```python
from build123d import *

# Parameters (mm, degrees)
SKETCH1_W           = 210
SKETCH1_H           = 439.61
BOSS_EXTRUDE1_DEPTH = 2
SKETCH2_W           = 210
SKETCH2_H           = 2
BOSS_EXTRUDE2_DEPTH = 20.32
FILLET1_R           = 1
FILLET2_R           = 1.5
SKETCH4_R           = 1.6
CUT_EXTRUDE1_DEPTH  = 1134.166859304


with BuildPart() as part:
    # Sketch1 → Boss-Extrude1 (new body)
    with BuildSketch(Plane(origin=(0, 0, 0), x_dir=(1, 0, 0), z_dir=(0, 1, 0))):
        with Locations((988.720815229, 75.734721456)):
            Rectangle(SKETCH1_W, SKETCH1_H)
    extrude(amount=BOSS_EXTRUDE1_DEPTH)

    # Sketch2 → Boss-Extrude2 (add)
    with BuildSketch(Plane.XZ):
        with Locations((988.720815229, 143.070278544)):
            Rectangle(SKETCH2_W, SKETCH2_H)
        with Locations((988.720815229, -294.539721456)):
            Rectangle(SKETCH2_W, SKETCH2_H)
    extrude(amount=BOSS_EXTRUDE2_DEPTH)

    # Fillet1
    fillet1_edges = [part.edges().sort_by_distance(p)[0] for p in [
        (988.720815229, 0, 142.070278544),
        (988.720815229, 0, -293.539721456),
    ]]
    fillet(fillet1_edges, radius=FILLET1_R)

    # Fillet2
    fillet2_edges = [part.edges().sort_by_distance(p)[0] for p in [
        (988.720815229, 2, 144.070278544),
        (988.720815229, 2, -295.539721456),
    ]]
    fillet(fillet2_edges, radius=FILLET2_R)

    # Sketch4 → Cut-Extrude1 (cut, through all)
    with BuildSketch(Plane(origin=(0, 2, 0), x_dir=(1, 0, 0), z_dir=(0, 1, 0))):
        with Locations(Location((921.920815229, 214.039721456, 0), (0, 0, 270))):
            Circle(SKETCH4_R)
        with Locations(Location((921.920815229, 274.039721456, 0), (0, 0, 270))):
            Circle(SKETCH4_R)
        with Locations(Location((986.920815229, 234.750399575, 0), (0, 0, 270))):
            Circle(SKETCH4_R)
        with Locations(Location((986.920815229, 274.039721456, 0), (0, 0, 270))):
            Circle(SKETCH4_R)
        with Locations(Location((1010.309162877, 65.651373808, 0), (0, 0, 270))):
            Circle(SKETCH4_R)
        with Locations(Location((1010.309162877, 95.651373808, 0), (0, 0, 270))):
            Circle(SKETCH4_R)
        with Locations(Location((986.565606348, -21.848626192, 0), (0, 0, 270))):
            Circle(SKETCH4_R)
        with Locations(Location((959.065606348, -21.848626192, 0), (0, 0, 270))):
            Circle(SKETCH4_R)
        with Locations(Location((963.168146726, 43.151373808, 0), (0, 0, 270))):
            Circle(SKETCH4_R)
        with Locations(Location((921.565606348, 43.151373808, 0), (0, 0, 270))):
            Circle(SKETCH4_R)
        with Locations(Location((894.065606348, -34.348626192, 0), (0, 0, 270))):
            Circle(SKETCH4_R)
        with Locations(Location((894.065606348, 15.651373808, 0), (0, 0, 270))):
            Circle(SKETCH4_R)
        with Locations(Location((961.370669454, -59.263980407, 0), (0, 0, 270))):
            Circle(SKETCH4_R)
        with Locations(Location((945.453731167, -122.879875269, 0), (0, 0, 270))):
            Circle(SKETCH4_R)
        with Locations(Location((896.92248209, -74.348626192, 0), (0, 0, 270))):
            Circle(SKETCH4_R)
        with Locations(Location((1073.720815229, -60.736751011, 0), (0, 0, 270))):
            Circle(SKETCH4_R)
        with Locations(Location((985.453731167, -60.736751011, 0), (0, 0, 270))):
            Circle(SKETCH4_R)
        with Locations(Location((1073.720815229, -125.736751011, 0), (0, 0, 270))):
            Circle(SKETCH4_R)
        with Locations(Location((985.453731167, -125.736751011, 0), (0, 0, 270))):
            Circle(SKETCH4_R)
        with Locations(Location((1013.305977837, -13.343657344, 0), (0, 0, 270))):
            Circle(SKETCH4_R)
        with Locations(Location((1058.564216667, 12.786773537, 0), (0, 0, 270))):
            Circle(SKETCH4_R)
        with Locations(Location((996.746475218, 52.151079456, 0), (0, 0, 270))):
            Circle(SKETCH4_R)
        with Locations(Location((938.352910915, 174.501024052, 0), (0, 0, 270))):
            Circle(SKETCH4_R)
        with Locations(Location((998.456987316, 114.396947651, 0), (0, 0, 270))):
            Circle(SKETCH4_R)
        with Locations(Location((998.866251712, 205.91156481, 0), (0, 0, 270))):
            Circle(SKETCH4_R)
        with Locations(Location((1058.970328113, 145.807488409, 0), (0, 0, 270))):
            Circle(SKETCH4_R)
        with Locations(Location((1075.308219227, 106.361698083, 0), (0, 0, 270))):
            Circle(SKETCH4_R)
        with Locations(Location((1075.305408117, 46.781698149, 0), (0, 0, 270))):
            Circle(SKETCH4_R)
    extrude(amount=-CUT_EXTRUDE1_DEPTH, mode=Mode.SUBTRACT)


solid = part.part
```
Can you work these out from the model? Positions are in its coordinate system, mm. A direction names the side the tool comes from. Coordinates: 2 decimals unless noted, no trailing zeros. Loops run counter-clockwise (first coordinate to the right, second up) from the corner with the lowest first, then second, coordinate; pieces in that order, holes last. Notation, with made-up numbers: (26.25, 81.5) -> (55.25, 81.5) arc R22 cw to (55.25, 105.5) -> close; hole circle Ø10 at (13, 78.5). An arc over 180 degrees is marked (long way). Answer as a JSON object with one key per item and string values.
1) For P1, Ø6, axis at x = 928, z = -175.5, coming from the -Y side, with a flat end and sliding along its axis, tell me the tip position at first contact or that it passes through.
Results:
{"P1": "stops at y = 0"}
2) For faces 5 (the face through (1093.721, 1, -77)), 6 (the face through (987, 0, -79)), which set-ups out of +Z, -Z, +X, -X, +Y, -Y let a thin tool reach every point of the face, with its end or its side?
Results:
{"face 5": "+Z, -Z, +X, +Y, -Y", "face 6": "+X, -X, -Y"}
3) If I drill on line 1 (Z direction, x = 1075.5, y = -4.5); line 2 (Y direction, x = 905, z = -100), over which ranges is the centre line in solid material (lowest first)?
Results:
{"line 1": "z = -295.54 to -293.54, 142.07 to 144.07", "line 2": "y = 0 to 2"}
4) Imagine slicing it at B-B (x = 927.5). Please give me the cut outline in (y, z).
Results:
{"outline": "(-20.32, -295.54) -> (0.5, -295.54) arc R1.5 ccw to (2, -294.04) -> (2, 142.57) arc R1.5 ccw to (0.5, 144.07) -> (-20.32, 144.07) -> (-20.32, 142.07) -> (-1, 142.07) arc R1 cw to (0, 141.07) -> (0, -292.54) arc R1 cw to (-1, -293.54) -> (-20.32, -293.54) -> close"}
5) Thinking about a two-plate mould opening in Z: for faces 1 (the face through (883.721, 1, -77)), 2 (the face through (987, -11, -293.54)), 3 (the face through (987, -11, 142.07)), 4 (the face through (987, -10, 144.07)), which applies, pulls with the +Z half, pulls with the -Z half, needs draft (parallel to the pull), parting line crosses it, or undercut?
Results:
{"face 1": "needs draft", "face 2": "undercut", "face 3": "undercut", "face 4": "pulls with the +Z half"}
6) Imagine slicing it at A-A (y = -7.75). Please give me the cut outline in (x, z).
Results:
{"outline": "(883.72, -295.54) -> (1093.72, -295.54) -> (1093.72, -293.54) -> (883.72, -293.54) -> close; (883.72, 142.07) -> (1093.72, 142.07) -> (1093.72, 144.07) -> (883.72, 144.07) -> close"}
7) Imagine slicing it at C-C (z = -225.5). Please give me the cut outline in (x, y), then the cut area to 3 significant figures.
Results:
{"outline": "(883.72, 0) -> (1093.72, 0) -> (1093.72, 2) -> (883.72, 2) -> close", "area": "420 mm^2"}
